Autodesk Inventor part; units mm, degrees
ref_plane "YZ Plane" through (0, 0, 0) normal (1, 0, 0) x (0, 1, 0)
ref_plane "XZ Plane" through (0, 0, 0) normal (0, 1, 0) x (-1, 0, 0)
ref_plane "XY Plane" through (0, 0, 0) normal (0, 0, 1) x (1, 0, 0)
sketch "Sketch1" plane through (0, 0, 0) normal (1, 0, 0) x (0, 1, 0)
  line L0 (86.7421, 202.4836) -> (-14.8579, 202.4836)
  line L1 (-14.8579, 202.4836) -> (-14.8579, -0.7164)
  line L2 (-14.8579, -0.7164) -> (86.7421, -0.7164)
  line L3 (86.7421, -0.7164) -> (86.7421, 202.4836)
  point P0 (0, 0)
  dimension "d0" = 101.6
  dimension "d1" = 203.2
extrude "Extrusion1" add sketch "Sketch1" along normal blind 3.175
sketch "Sketch2" plane through (3.175, 0, 0) normal (1, 0, 0) x (0, 0, -1)
  line L0 (-202.4836, 86.7421) -> (-202.4836, -14.8579) construction
  line L1 (-202.4836, 35.9421) -> (-177.0836, 35.9421) construction
  line L2 (-177.0836, 35.9421) -> (-144.0636, 35.9421) construction
  circle A0 centre (-144.0636, 35.9421) radius 11.1125
  line L3 (-144.0636, 35.9421) -> (-103.4236, 35.9421) construction
  line L4 (-103.4236, 35.9421) -> (-62.7836, 35.9421) construction
  circle A1 centre (-103.4236, 35.9421) radius 11.1125
  circle A2 centre (-62.7836, 35.9421) radius 14.2875
  circle A3 centre (-177.0836, 35.9421) radius 9.525
  point P0 (0, 0)
  dimension "d4" = 25.4
  dimension "d5" = 33.02
  dimension "d7" = 22.225
  dimension "d8" = 40.64
  dimension "d9" = 40.64
  dimension "d10" = 22.225
  dimension "d11" = 28.575
  dimension "d14" = 19.05
extrude "Extrusion2" cut sketch "Sketch2" against normal blind 12.7
sketch "Sketch3" plane through (0, 0, 0) normal (-1, 0, 0) x (0, 0, 1)
  circle A0 centre (177.0836, 35.9421) radius 9.525
  circle A1 centre (177.0836, 61.3421) radius 2.0193
  circle A2 centre (177.0836, 10.5421) radius 2.0193
  line L0 (177.0836, 61.3421) -> (177.0836, 10.5421) construction
  point P0 (0, 0)
  dimension "d17" = 4.0386
  dimension "d18" = 4.0386
extrude "Extrusion3" cut sketch "Sketch3" against normal blind 25.4 contours A1 | A2
properties part number "ARm Gearbox Plate"
Work out the finished part from the listing and answer in its coordinate system (mm). Give positions to 0.01 mm unless a question says otherwise; leave off trailing zeros. Loops run counter-clockwise (first coordinate to the right, second up) from the corner with the lowest first, then second, coordinate; pieces in that order, holes last. Notation, with made-up numbers: (29.5, 32.25) - (74.5, 32.25) arc R15 cw to (74.5, 44.25) - close; hole circle Ø8 at (47.25, -30.75). An arc over 180 degrees is marked (long way). Answer in a Markdown table with one row per item.
(1) Section A-A (z = 107) is taken. Give the vertices of the cut face in (x, y) (3 decimals).
Results list:
| item | result |
|---|---|
| outline | (0, -14.858) - (3.175, -14.858) - (3.175, 25.421) - (0, 25.421) - close; (0, 46.463) - (3.175, 46.463) - (3.175, 86.742) - (0, 86.742) - close |
(2) Consider L1, parallel to Y at x = 2.9, z = 140; L2, parallel to Z at x = 2.15, y = 31; L3, parallel to Y at x = 2.65, z = 148.5. Determine where each line is inside the solid, lowest interval first. Write a range as [from, to].
Results list:
| item | result |
|---|---|
| L1 | y = [-14.86, 25.6], [46.28, 86.74] |
| L2 | z = [-0.72, 49.38], [76.19, 93.47], [113.38, 134.11], [154.02, 168.94], [185.23, 202.48] |
| L3 | y = [-14.86, 25.75], [46.13, 86.74] |
(3) Flat-ended cylindrical pins translate along their axes: pin 1 Ø23 at (y, z) = (35.94, 62.78) entering from +X; pin 2 Ø1 at (y, z) = (72, 88) entering from -X. Find the tip coordinate at first contact, or state that the pin passes through.
Results list:
| item | result |
|---|---|
| pin 1 | passes through |
| pin 2 | stops at x = 0 |
(4) Section C-C (z = 75) is taken. Give the vertices of the cut face in (x, y) (3 decimals), and give its area (3 significant figures).
Results list:
| item | result |
|---|---|
| outline | (0, -14.858) - (3.175, -14.858) - (3.175, 28.533) - (0, 28.533) - close; (0, 43.351) - (3.175, 43.351) - (3.175, 86.742) - (0, 86.742) - close |
| area | 276 mm² |
(5) For a pull along Y with two mould halves and no side action, classify faces 1 (the face through (1.57, 11.15, 179.01)), 2 (the face through (0, 24, 102)) as pulls with the +Y half, pulls with the -Y half, needs draft (parallel to the pull), parting line crosses it, or undercut.
Results list:
| item | result |
|---|---|
| face 1 | undercut |
| face 2 | needs draft |
(6) Section B-B (x = 2.15) is taken. State how many separate pieces and enclosed holes the cut face has, and give its area (3 significant figures).
Results list:
| item | result |
|---|---|
| separate pieces | 1 |
| enclosed holes | 6 |
| area | 18,900 mm² |
